Verification items for the finished model (mm, model axes). A direction names the side the tool comes from. Round coordinates to 2 decimals unless told otherwise and drop trailing zeros. Order: outer loops, then holes, each group sorted by start corner. A loop starts at its lowest first (then second) coordinate and runs counter-clockwise, first axis right, second up. Notation, with made-up numbers: M 33,33.25 L 55,33.25 A9 ccw 55,45.25 Z; hole C 34.5,2.25 d9. An arc over 180 degrees is marked long. Return JSON: item names as keys, results as strings. Group by question number.
from build123d import *

# Parameters (mm, degrees)
SALIENTE_EXTRUIR1_DEPTH = 12.7
CROQUIS1_4_OUTSIDE_W    = 75.96
CROQUIS1_4_OUTSIDE_H    = 75.96
CROQUIS1_4_OUTSIDE_R    = 1.693796282
CORTAR_EXTRUIR1_DEPTH   = 29.7
CROQUIS2_R              = 19
CORTAR_EXTRUIR2_DEPTH   = 2
CROQUIS3_R              = 10.75
CORTAR_EXTRUIR3_DEPTH   = 43.043013688
CROQUIS4_R              = 5.5
CORTAR_EXTRUIR4_DEPTH   = 10
CROQUIS6_R              = 3.15
CORTAR_EXTRUIR5_DEPTH   = 42.870335561


with BuildPart() as part:
    # Croquis1 → Saliente-Extruir1 (new body)
    with BuildSketch(Plane(origin=(0, 0, 0), x_dir=(1, 0, 0), z_dir=(0, 1, 0))):
        with BuildLine():
            Line((-27.25, -28.75), (27.25, -28.75))
            ThreePointArc((27.25, -28.75), (28.310660172, -28.310660172), (28.75, -27.25))
            Line((28.75, -27.25), (28.75, 27.25))
            ThreePointArc((28.75, 27.25), (28.310660172, 28.310660172), (27.25, 28.75))
            Line((27.25, 28.75), (-27.25, 28.75))
            ThreePointArc((-27.25, 28.75), (-28.310660172, 28.310660172), (-28.75, 27.25))
            Line((-28.75, 27.25), (-28.75, -27.25))
            ThreePointArc((-28.75, -27.25), (-28.310660172, -28.310660172), (-27.25, -28.75))
        make_face()
    extrude(amount=SALIENTE_EXTRUIR1_DEPTH)

    # Croquis1_4 outside → Cortar-Extruir1 (cut)
    # profile 1 of 5: a face of its own
    with BuildSketch(Plane(origin=(0, 0, 0), x_dir=(1, 0, 0), z_dir=(0, 1, 0))):
        Rectangle(CROQUIS1_4_OUTSIDE_W, CROQUIS1_4_OUTSIDE_H)
        with BuildLine():
            Line((-27.25, -28.75), (27.25, -28.75))
            ThreePointArc((27.25, -28.75), (28.310660172, -28.310660172), (28.75, -27.25))
            Line((28.75, -27.25), (28.75, 27.25))
            ThreePointArc((28.75, 27.25), (28.310660172, 28.310660172), (27.25, 28.75))
            Line((27.25, 28.75), (-27.25, 28.75))
            ThreePointArc((-27.25, 28.75), (-28.310660172, 28.310660172), (-28.75, 27.25))
            Line((-28.75, 27.25), (-28.75, -27.25))
            ThreePointArc((-28.75, -27.25), (-28.310660172, -28.310660172), (-27.25, -28.75))
        make_face(mode=Mode.SUBTRACT)
    # profile 2 of 5: a face of its own
    with BuildSketch(Plane(origin=(0, 0, 0), x_dir=(1, 0, 0), z_dir=(0, 1, 0))):
        with Locations(Location((-23.75, 23.75, 0), (0, 0, 270))):
            Circle(CROQUIS1_4_OUTSIDE_R)
    # profile 3 of 5: a face of its own
    with BuildSketch(Plane(origin=(0, 0, 0), x_dir=(1, 0, 0), z_dir=(0, 1, 0))):
        with Locations(Location((23.75, 23.75, 0), (0, 0, 90))):
            Circle(CROQUIS1_4_OUTSIDE_R)
    # profile 4 of 5: a face of its own
    with BuildSketch(Plane(origin=(0, 0, 0), x_dir=(1, 0, 0), z_dir=(0, 1, 0))):
        with Locations(Location((23.75, -23.75, 0), (0, 0, 270))):
            Circle(CROQUIS1_4_OUTSIDE_R)
    # profile 5 of 5: a face of its own
    with BuildSketch(Plane(origin=(0, 0, 0), x_dir=(1, 0, 0), z_dir=(0, 1, 0))):
        with Locations(Location((-23.75, -23.75, 0), (0, 0, 90))):
            Circle(CROQUIS1_4_OUTSIDE_R)
    extrude(amount=CORTAR_EXTRUIR1_DEPTH, mode=Mode.SUBTRACT)

    # Croquis2 → Cortar-Extruir2 (cut)
    with BuildSketch(Plane.XZ):
        with Locations(Location((0, 0, 0), (0, 0, 270))):
            Circle(CROQUIS2_R)
    extrude(amount=-CORTAR_EXTRUIR2_DEPTH, mode=Mode.SUBTRACT)

    # Croquis3 → Cortar-Extruir3 (cut, through all)
    with BuildSketch(Plane.XZ.offset(-2)):
        with Locations(Location((0, 0, 0), (0, 0, 270))):
            Circle(CROQUIS3_R)
    extrude(amount=-CORTAR_EXTRUIR3_DEPTH, mode=Mode.SUBTRACT)

    # Croquis4 → Cortar-Extruir4 (cut)
    with BuildSketch(Plane.XZ):
        with Locations(Location((22.55, 0, 0), (0, 0, 270))):
            Circle(CROQUIS4_R)
        with Locations(Location((0, -22.55, 0), (0, 0, 270))):
            Circle(CROQUIS4_R)
        with Locations(Location((-22.55, 0, 0), (0, 0, 270))):
            Circle(CROQUIS4_R)
        with Locations(Location((0, 22.55, 0), (0, 0, 270))):
            Circle(CROQUIS4_R)
    extrude(amount=-CORTAR_EXTRUIR4_DEPTH, mode=Mode.SUBTRACT)

    # Croquis6 → Cortar-Extruir5 (cut, through all)
    with BuildSketch(Plane.XZ.offset(-10)):
        with Locations(Location((22.55, 0, 0), (0, 0, 270))):
            Circle(CROQUIS6_R)
        with Locations(Location((0, -22.55, 0), (0, 0, 270))):
            Circle(CROQUIS6_R)
        with Locations(Location((-22.55, 0, 0), (0, 0, 270))):
            Circle(CROQUIS6_R)
        with Locations(Location((0, 22.55, 0), (0, 0, 270))):
            Circle(CROQUIS6_R)
    extrude(amount=-CORTAR_EXTRUIR5_DEPTH, mode=Mode.SUBTRACT)


solid = part.part
1. Go/stop test with flat-tipped pins: pin 1 (5 mm diameter, centred on x = -21, z = -1, fed in from -Y); pin 2 (2.5 mm diameter, centred on x = -23.75, z = -23.75, fed in from -Y). Record where each tip stops, or that it passes through.
2. Draft check along Z on faces 3 (the face through (-19.427, 11.331, 0.41)), 4 (the face through (0, 6, -28.75)), 5 (the face through (0, 6, 28.75)). Enter one of: +Z half, -Z half, draft (parallel to the pull), parting line (faces both ways), or undercut.
3. Cross-section at A-A (z = 0). Enter the section's corners in (x, y).
4. Thickness scan on line 1 along X through (y, z) = (11.8, 0); line 2 along X through (y, z) = (3.75, 0); line 3 along Z through (x, y) = (-25, 10.75). Record the ranges inside material, lowest first. Write a range as from..to.
5. Cross-section at C-C (y = 4.5). Give the number of separate pieces and of enclosed holes in the cut face, plus the area to 3 significant figures.
6. Access from +Z, -Z, +X, -X, +Y, -Y to the whole of each face (thin tool, end or side, straight path). Record for faces 1 (the face through (7.27, 7.28, 7.92)), 2 (the face through (-13.54, 0.99, -13.33)).
7. Cross-section at B-B (x = 10). Enter the section's corners in (y, z), plus the area to 3 significant figures.
8. Cross-section at D-D (x = 23.75). Enter the section's corners in (y, z), plus the area to 3 significant figures.
Computed:
{
 "1": {"pin 1": "stops at y = 10", "pin 2": "passes through"},
 "2": {"face 3": "undercut", "face 4": "-Z half", "face 5": "+Z half"},
 "3": {"outline": "M -28.75,0 L -28.05,0 L -28.05,10 L -25.7,10 L -25.7,12.7 L -28.75,12.7 Z; M -19.4,10 L -17.05,10 L -17.05,2 L -10.75,2 L -10.75,12.7 L -19.4,12.7 Z; M 10.75,2 L 17.05,2 L 17.05,10 L 19.4,10 L 19.4,12.7 L 10.75,12.7 Z; M 25.7,10 L 28.05,10 L 28.05,0 L 28.75,0 L 28.75,12.7 L 25.7,12.7 Z"},
 "4": {"line 1": "x = -28.75..-25.7, -19.4..-10.75, 10.75..19.4, 25.7..28.75", "line 2": "x = -28.75..-28.05, -17.05..-10.75, 10.75..17.05, 28.05..28.75", "line 3": "z = -28.75..-24.89, -22.61..-1.98, 1.98..22.61, 24.89..28.75"},
 "5": {"separate pieces": "1", "enclosed holes": "9", "area": "2,530 mm²"},
 "6": {"face 1": "+Y, -Y", "face 2": "-Y"},
 "7": {"outline": "M 0,-28.75 L 12.7,-28.75 L 12.7,-3.94 L 2,-3.94 L 2,-16.16 L 0,-16.16 Z; M 0,16.16 L 2,16.16 L 2,3.94 L 12.7,3.94 L 12.7,28.75 L 0,28.75 Z", "area": "581 mm²"},
 "8": {"outline": "M 0,-28.75 L 12.7,-28.75 L 12.7,-25.44 L 0,-25.44 Z; M 0,-22.06 L 12.7,-22.06 L 12.7,-2.91 L 10,-2.91 L 10,-5.37 L 0,-5.37 Z; M 0,5.37 L 10,5.37 L 10,2.91 L 12.7,2.91 L 12.7,22.06 L 0,22.06 Z; M 0,25.44 L 12.7,25.44 L 12.7,28.75 L 0,28.75 Z", "area": "521 mm²"}
}
